Check sheet for the drawn part. Datum: minimum x, y, z corner. Units: mm. A direction names the side the tool comes from. Give positions to 0.01 mm unless a question says otherwise; leave off trailing zeros. Loops run counter-clockwise (first coordinate to the right, second up) from the corner with the lowest first, then second, coordinate; pieces in that order, holes last. Notation, with made-up numbers: M 46,24.5 L 89,24.5 A19 cw 89,34.5 Z; hole C 78.5,80.5 d9. An arc over 180 degrees is marked long. Write each question's results on one line, items separated by ' | '. Start each with the question number.
1. Go/stop test with flat-tipped pins: pin 1 (1.5 mm diameter, centred on x = 47.5, y = 52.5, fed in from -Z); pin 2 (0.9 mm diameter, centred on x = 11.5, z = 18, fed in from -Y); pin 3 (4 mm diameter, centred on y = 17, z = 14, fed in from -X). Record where each tip stops, or that it passes through.
2. Sectioned sample at C-C on x = 28. Record the cut outline in (y, z), and give its area (3 significant figures).
3. Sectioned sample at B-B on z = 27.5. Give the number of separate pieces and of enclosed holes in the cut face, and give its area (3 significant figures).
4. Draft check along X on the marked faces 4, 5 and 6. Enter one of: pulls with the +X half, pulls with the -X half, needs draft (parallel to the pull), parting line crosses it, or undercut.
5. Material ranges on line 1 along Y through (x, z) = (3.5, 27); line 2 along X through (y, z) = (28, 31.5); line 3 along Y through (x, z) = (12.5, 13.5), recorded low to high.
6. Sectioned sample at D-D on y = 49. Record the cut outline in (x, z).
7. Sectioned sample at A-A on y = 67. Record the cut outline in (x, z).
8. Tool access check on the marked faces 1, 2 and 3. Record the directions out of +Z, -Z, +X, -X, +Y, -Y that give a thin tool (end or side, any length) a straight path to the whole face; none if there is none.
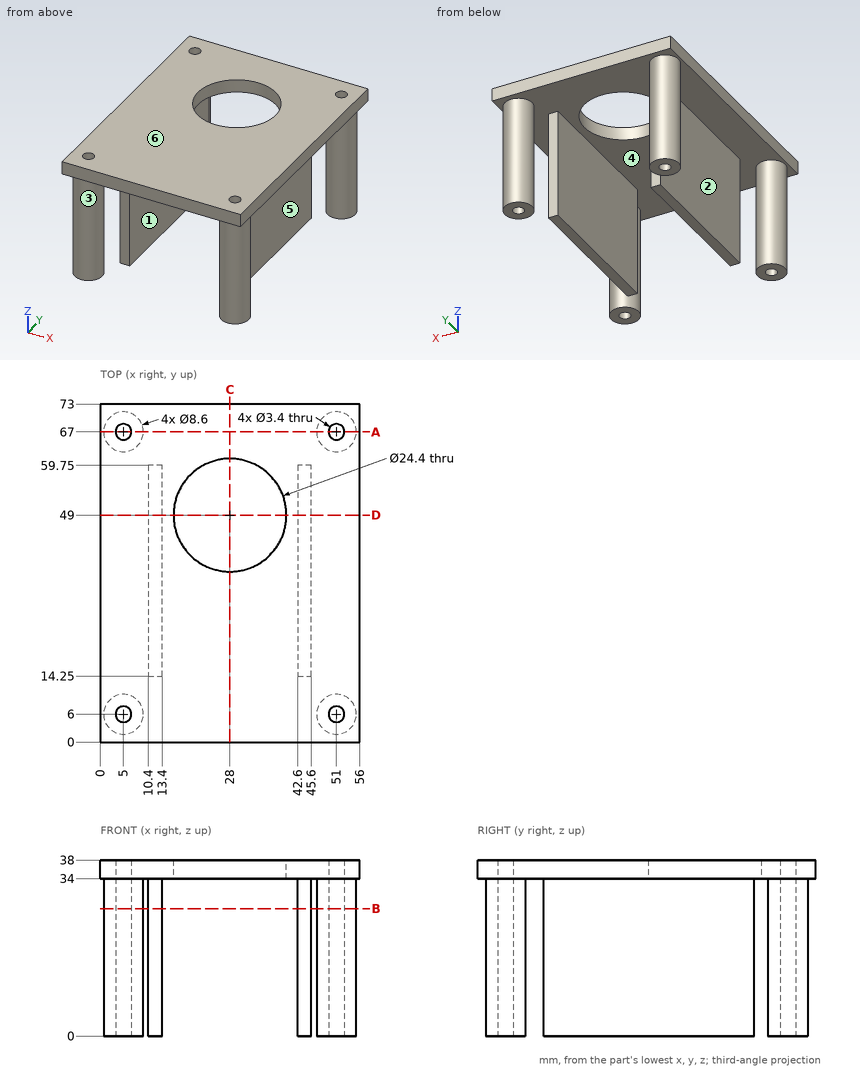
Output values:
1) pin 1: z = 34 | pin 2: y = 14.25 | pin 3: x = 10.4
2) outline: M 0,34 L 36.8,34 L 36.8,38 L 0,38 Z; M 61.2,34 L 73,34 L 73,38 L 61.2,38 Z | area: 194 mm2
3) separate pieces: 6 | enclosed holes: 4 | area: 469 mm2
4) face 4: undercut | face 5: pulls with the +X half | face 6: needs draft
5) line 1: 1.97 to 5.2, 6.8 to 10.03, 62.97 to 66.2, 67.8 to 71.03 | line 2: 10.4 to 13.4, 42.6 to 45.6 | line 3: 14.25 to 59.75
6) outline: M 0,34 L 10.4,34 L 10.4,0 L 13.4,0 L 13.4,34 L 15.8,34 L 15.8,38 L 0,38 Z; M 40.2,34 L 42.6,34 L 42.6,0 L 45.6,0 L 45.6,34 L 56,34 L 56,38 L 40.2,38 Z
7) outline: M 0,34 L 0.7,34 L 0.7,0 L 3.3,0 L 3.3,38 L 0,38 Z; M 6.7,0 L 9.3,0 L 9.3,34 L 46.7,34 L 46.7,0 L 49.3,0 L 49.3,38 L 6.7,38 Z; M 52.7,0 L 55.3,0 L 55.3,34 L 56,34 L 56,38 L 52.7,38 Z
8) face 1: -Z, +Y, -Y | face 2: -Z, -X, +Y, -Y | face 3: -Z
